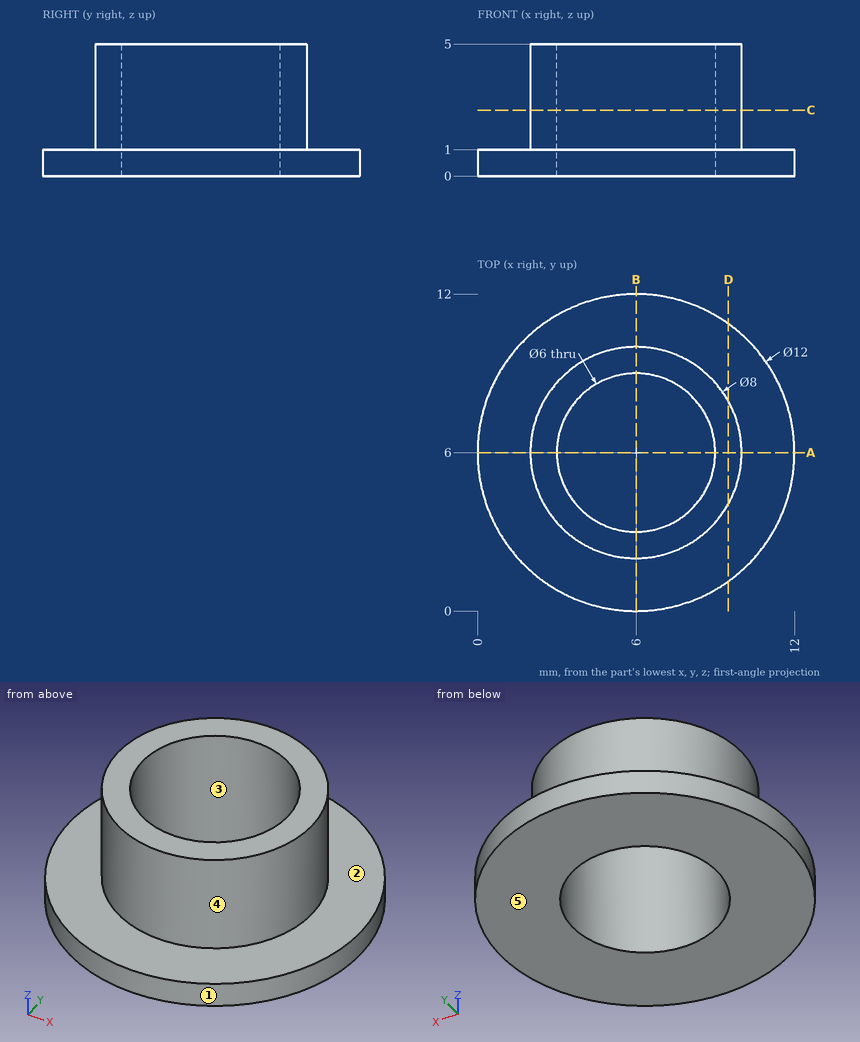
Part print with two shaded views. Sizes in mm from the minimum x, y, z corner. A direction names the side the tool comes from. Round coordinates to 2 decimals unless told otherwise and drop trailing zeros. Loops run counter-clockwise (first coordinate to the right, second up) from the corner with the lowest first, then second, coordinate; pieces in that order, holes last. Notation, with made-up numbers: M 43.25,20.5 L 101.25,20.5 A16 ccw 101.25,32.5 Z; hole C 61.25,-17 d5. An arc over 180 degrees is marked long. Put each result on its own line as item: value. Start each with the question number.
Item 1: Cut at A-A (y = 6). List the corners of the cut face in (x, z), then the cut area to 3 significant figures.
Item 2: Drop flat-ended pins along their axis: P1, Ø6, axis at x = 9, y = 9.5, coming from the +Z side; P2, Ø2, axis at x = 5.5, y = 4.5, coming from the -Z side. Give the stop position or say it passes through.
Item 3: Drill centre lines: line 1 along Y through (x, z) = (6, 1.45); line 2 along Y through (x, z) = (5, 1.3); line 3 along X through (y, z) = (6.25, 1.3). Where is each one in solid material? Low to high.
Item 4: 3-axis set-ups, long thin cutter, end or side, ignore diameter. For the marked faces 1 and 2: which of +Z, -Z, +X, -X, +Y, -Y reach the whole face in a straight line?
Item 5: Mould opens along X. For the marked faces 3, 4 and 5 say: released by +X, released by -X, zero draft, split by the parting line, or undercut.
Item 6: Cut at D-D (x = 9.5). List the corners of the cut face in (y, z).
Item 7: Cut at C-C (z = 2.5). List the corners of the cut face in (x, y).
Answer block:
1. outline: M 0,0 L 3,0 L 3,5 L 2,5 L 2,1 L 0,1 Z; M 9,0 L 12,0 L 12,1 L 10,1 L 10,5 L 9,5 Z
1. area: 14.0 mm2
2. P1: z = 5
2. P2: through
3. line 1: 2 to 3, 9 to 10
3. line 2: 2.13 to 3.17, 8.83 to 9.87
3. line 3: 2.01 to 3.01, 8.99 to 9.99
4. face 1: +Z, -Z
4. face 2: +Z
5. face 3: undercut
5. face 4: split by the parting line
5. face 5: zero draft
6. outline: M 1.13,0 L 10.87,0 L 10.87,1 L 7.94,1 L 7.94,5 L 4.06,5 L 4.06,1 L 1.13,1 Z
7. outline: C 6,6 d8; hole C 6,6 d6
